Drawing for the job (mm, zero at the part's lowest x, y, z). A direction names the side the tool comes from. Give positions to 0.01 mm unless a question says otherwise; leave off trailing zeros. Order: outer loops, then holes, each group sorted by start corner. A loop starts at its lowest first (then second) coordinate and runs counter-clockwise, first axis right, second up. Notation, with made-up numbers: (21.25, 55.5) - (54.25, 55.5) arc R7 ccw to (54.25, 59.5) - close; hole circle Ø10 at (31, -14.75). An arc over 180 degrees is marked (long way). Use a Markdown table: item, result. Add a question column.
(1) Which spindle directions (+Z, -Z, +X, -X, +Y, -Y) get a long thin tool onto all of the face, cutting with end or side? Do the marked faces 4, 5, 6, 7 and 8. Say none if no direction does.
(2) Slice it at A-A (x = 24). Write the cut outline in (y, z).
(3) Slice it at C-C (y = 13.25). Write the cut outline in (x, z), then the cut area to 3 significant figures.
(4) Wall check: line 1 (Z direction, x = 24, y = 13.1); line 2 (X direction, y = 8, z = 5); line 3 (Z direction, x = 26, y = 5.25). Give the ranges that are in metal, low to high.
(5) Slice it at D-D (y = 6). Write the cut outline in (x, z).
(6) Flat gauge pins, fed straight in: pin 1 (4.5 mm diameter, centred on x = 14.5, y = 9, fed in from +Z); pin 2 (3.5 mm diameter, centred on y = 13.5, z = 38.5, fed in from -X); pin 3 (2 mm diameter, centred on x = 8.5, y = 11.5, fed in from -Z). Where does each tip first touch, or does it go through?
(7) Slice it at B-B (z = 44). Write the cut outline in (x, y).
(8) Mould opens along Z. For the marked faces 1, 2 and 3 say: +Z half, -Z half, draft (parallel to the pull), parting line (faces both ways), or undercut.
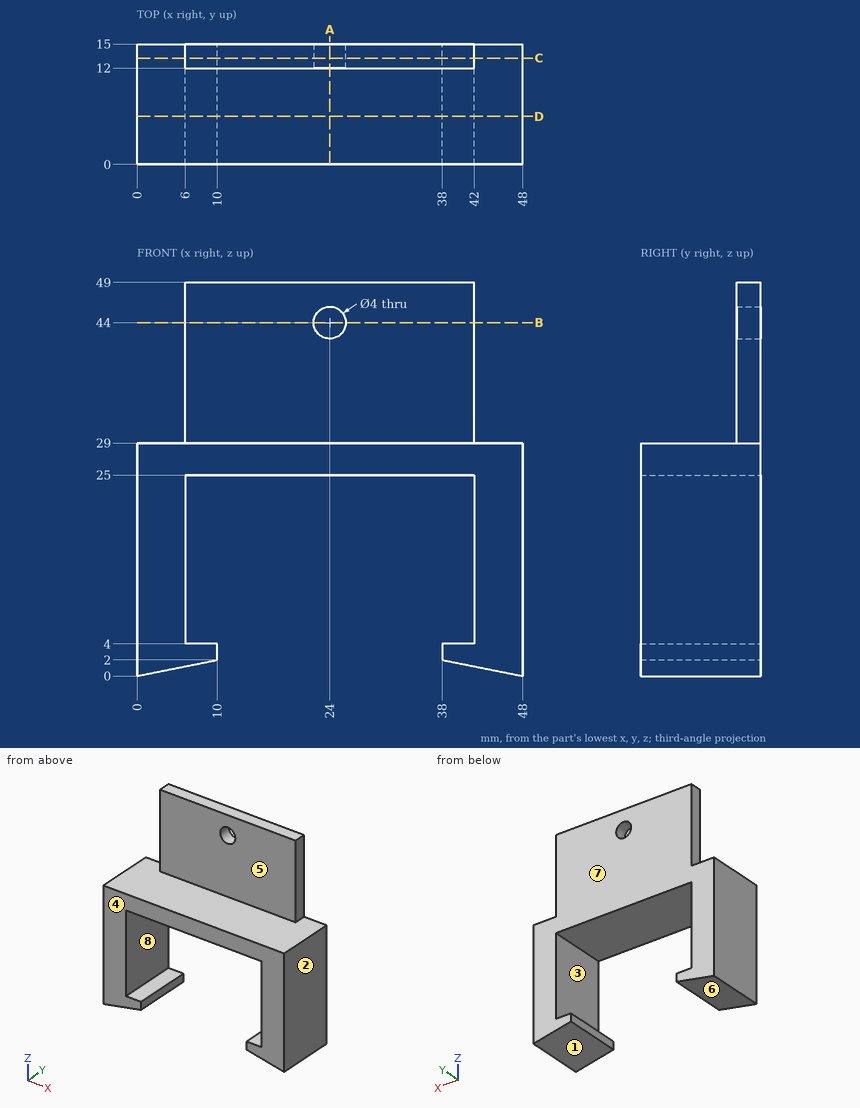
Solution:
| question | item | result |
|---|---|---|
| 1 | face 4 | +Z, -Z, +X, -X, -Y |
| 1 | face 5 | +Z, +X, -X, -Y |
| 1 | face 6 | -Z, +Y, -Y |
| 1 | face 7 | +Z, -Z, +X, -X, +Y |
| 1 | face 8 | +Y, -Y |
| 2 | outline | (0, 25) - (15, 25) - (15, 42) - (12, 42) - (12, 29) - (0, 29) - close; (12, 46) - (15, 46) - (15, 49) - (12, 49) - close |
| 3 | outline | (0, 0) - (10, 2) - (10, 4) - (6, 4) - (6, 25) - (42, 25) - (42, 4) - (38, 4) - (38, 2) - (48, 0) - (48, 29) - (42, 29) - (42, 49) - (6, 49) - (6, 29) - (0, 29) - close; hole circle Ø4 at (24, 44) |
| 3 | area | 1,210 mm2 |
| 4 | line 1 | 25 to 42, 46 to 49 |
| 4 | line 2 | 0 to 6, 42 to 48 |
| 4 | line 3 | 25 to 29 |
| 5 | outline | (0, 0) - (10, 2) - (10, 4) - (6, 4) - (6, 25) - (42, 25) - (42, 4) - (38, 4) - (38, 2) - (48, 0) - (48, 29) - (0, 29) - close |
| 6 | pin 1 | z = 29 |
| 6 | pin 2 | x = 6 |
| 6 | pin 3 | z = 1.5 |
| 7 | outline | (6, 12) - (22, 12) - (22, 15) - (6, 15) - close; (26, 12) - (42, 12) - (42, 15) - (26, 15) - close |
| 8 | face 1 | -Z half |
| 8 | face 2 | draft |
| 8 | face 3 | undercut |
